Verification items for this drawing (mm, ordinates from the low corner). A direction names the side the tool comes from. Round coordinates to 2 decimals unless told otherwise and drop trailing zeros. Write each loop counter-clockwise with the first axis right and the second up, starting at its lowest first coordinate (ties: lowest second). Pieces come first, ordered by that corner, then holes. Notation, with made-up numbers: (-28.5, -32.5) -> (-16.5, -32.5) arc R24 cw to (-16.5, -16.5) -> close; hole circle Ø3 at (-4.5, 36). An arc over 180 degrees is marked (long way). Put each result on its own line as item: value. Start each with the question number.
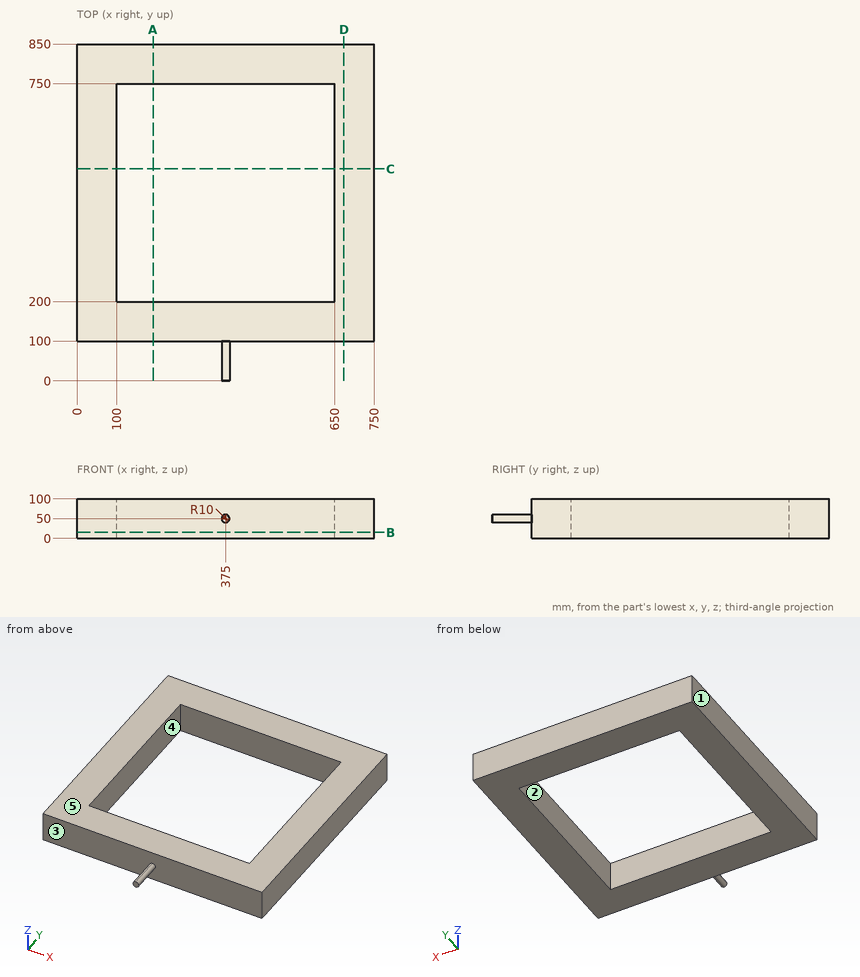
(1) Sectioned sample at C-C (y = 535). Record the cut outline in (x, z), and give its area (3 significant figures).
(2) Set-up check for the marked faces 4 and 5: record each of +Z, -Z, +X, -X, +Y, -Y from which the full face is reachable in a straight line by a thin tool's end or side.
(3) Material ranges on L1, parallel to Y at x = 181, z = 26; L2, parallel to X at y = 386.5, z = 75.5; L3, parallel to Y at x = 84, z = 67.5, recorded low to high. Write a range as from..to.
(4) Go/stop test with a flat-tipped pin: pin 1 Ø3 at (x, z) = (562, 47) entering from -Y. Record where the tip stops, or that it passes through.
(5) Sectioned sample at B-B (z = 15.5). Record the cut outline in (x, y).
(6) Sectioned sample at A-A (x = 192). Record the cut outline in (y, z), and give its area (3 significant figures).
(7) Mould release check, pull along Y, two halves, no side actions. Record for the marked faces 1, 2 and 3: +Y half, -Y half, draft (parallel to the pull), parting line (faces both ways), or undercut.
(8) Sectioned sample at D-D (x = 673.5). Record the cut outline in (y, z), and give its area (3 significant figures).
Found:
1. outline: (0, 0) -> (100, 0) -> (100, 100) -> (0, 100) -> close; (650, 0) -> (750, 0) -> (750, 100) -> (650, 100) -> close
1. area: 20,000 mm2
2. face 4: +Z, -Z
2. face 5: +Z, +X, -X, +Y, -Y
3. L1: 100..200, 750..850
3. L2: 0..100, 650..750
3. L3: 100..850
4. pin 1: y = 100
5. outline: (0, 100) -> (750, 100) -> (750, 850) -> (0, 850) -> close; hole (100, 200) -> (650, 200) -> (650, 750) -> (100, 750) -> close
6. outline: (100, 0) -> (200, 0) -> (200, 100) -> (100, 100) -> close; (750, 0) -> (850, 0) -> (850, 100) -> (750, 100) -> close
6. area: 20,000 mm2
7. face 1: draft
7. face 2: undercut
7. face 3: -Y half
8. outline: (100, 0) -> (850, 0) -> (850, 100) -> (100, 100) -> close
8. area: 75,000 mm2
